Here's how the part is built. I have some questions about the finished solid (model axes, mm). Face numbers are marked on the shaded views. Round coordinates to 2 decimals unless told otherwise and drop trailing zeros. Loops run counter-clockwise (first coordinate to the right, second up) from the corner with the lowest first, then second, coordinate; pieces in that order, holes last. Notation, with made-up numbers: (24.5, -14) - (53.5, -14) arc R35 ccw to (53.5, 19) - close; hole circle Ø11 at (50.25, 32). An arc over 180 degrees is marked (long way). Answer as a JSON object with one key per item and string values. Group by question number.
1) If I drill on line 1 along X through (y, z) = (0.25, -11); line 2 along Y through (x, z) = (5.75, 13); line 3 along Y through (x, z) = (2, -17), over which ranges is the centre line in solid material (lowest first)? Write a range as [from, to].
2) I want a section at D-D, the plane z = 17.5. Please give me the cut outline in (x, y).
3) Will these pins go through, and if not, where does the flat tip stop? P1, Ø1.2, axis at x = 0, z = -11.25, coming from the +Y side; P2, Ø3, axis at x = 0, y = -1.5, coming from the -Z side; P3, Ø8, axis at y = 5.5, z = 14.5, coming from the +X side; P4, Ø1.5, axis at y = 5.5, z = 7, coming from the +X side.
4) I want a section at C-C, the plane x = 3.25. Please give me the cut outline in (y, z).
5) If we mould it in two halves opening along X, with no side actions, what happens to the marked faces 1, 2 and 3? For each: pulls with the +X half, pulls with the -X half, needs draft (parallel to the pull), parting line crosses it, or undercut.
6) I want a section at B-B, the plane z = 0. Please give me the cut outline in (x, y), then the cut area to 3 significant figures.
7) I want a section at A-A, the plane x = 0. Please give me the cut outline in (y, z).
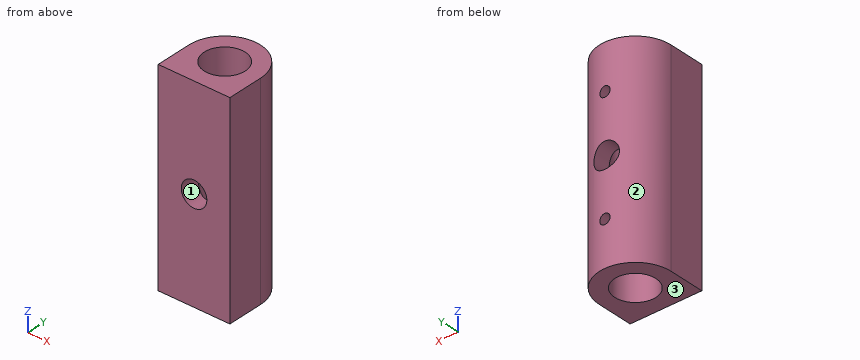
from build123d import *

# Parameters (mm, degrees)
SKETCH1_R           = 4
BOSS_EXTRUDE1_DEPTH = 20
SKETCH2_R           = 2.5
CUT_EXTRUDE1_DEPTH  = 26.396850198
SKETCH3_R           = 1
CUT_EXTRUDE2_DEPTH  = 23.315913757


with BuildPart() as part:
    # Sketch1 → Boss-Extrude1 (new, symmetric)
    with BuildSketch(Plane.XY):
        with BuildLine():
            Line((-7, 0), (-7, -7))
            Line((-7, -7), (7, -7))
            Line((7, -7), (7, 0))
            ThreePointArc((7, 0), (0, 7), (-7, 0))
        make_face()
        Circle(SKETCH1_R, mode=Mode.SUBTRACT)
    extrude(amount=BOSS_EXTRUDE1_DEPTH, both=True)

    # Sketch2 → Cut-Extrude1 (cut, through all)
    with BuildSketch(Plane(origin=(0, -7, 0), x_dir=(-1, 0, 0), z_dir=(0, -1, 0))):
        with Locations(Location((0, 0, 0), (0, 0, 180))):
            Circle(SKETCH2_R)
    extrude(amount=-CUT_EXTRUDE1_DEPTH, mode=Mode.SUBTRACT)

    # Sketch3 → Cut-Extrude2 (cut, through all)
    with BuildSketch(Plane(origin=(0, 0, 0), x_dir=(1, 0, 0), z_dir=(0, 1, 0))):
        with Locations(Location((0, 11.25, 0), (0, 0, 90))):
            Circle(SKETCH3_R)
        with Locations(Location((0, -11.25, 0), (0, 0, 90))):
            Circle(SKETCH3_R)
    extrude(amount=CUT_EXTRUDE2_DEPTH, mode=Mode.SUBTRACT)


solid = part.part
Outcome:
{
 "1": {"line 1": "[-7, -3.99], [3.99, 7]", "line 2": "[-7, 3.99]", "line 3": "[-7, -3.46], [3.46, 6.71]"},
 "2": {"outline": "(-7, -7) - (7, -7) - (7, 0) arc R7 ccw to (-7, 0) - close; hole circle Ø8 at (0, 0)"},
 "3": {"P1": "y = -3.95", "P2": "through", "P3": "x = 6.84", "P4": "x = 5.14"},
 "4": {"outline": "(-7, -20) - (-2.33, -20) - (-2.33, 20) - (-7, 20) - close; (2.33, -20) - (6.2, -20) - (6.2, 20) - (2.33, 20) - close"},
 "5": {"face 1": "undercut", "face 2": "parting line crosses it", "face 3": "needs draft"},
 "6": {"outline": "(-7, -7) - (-2.5, -7) - (-2.5, -3.12) arc R4 cw to (-2.5, 3.12) - (-2.5, 6.54) arc R7 ccw to (-7, 0) - close; (2.5, -7) - (7, -7) - (7, 0) arc R7 ccw to (2.5, 6.54) - (2.5, 3.12) arc R4 cw to (2.5, -3.12) - close", "area": "92.7 mm^2"},
 "7": {"outline": "(-7, -20) - (-4, -20) - (-4, -2.5) - (-7, -2.5) - close; (-7, 2.5) - (-4, 2.5) - (-4, 20) - (-7, 20) - close; (4, -20) - (7, -20) - (7, -12.25) - (4, -12.25) - close; (4, -10.25) - (7, -10.25) - (7, -2.5) - (4, -2.5) - close; (4, 2.5) - (7, 2.5) - (7, 10.25) - (4, 10.25) - close; (4, 12.25) - (7, 12.25) - (7, 20) - (4, 20) - close"}
}
